Verification items for the finished model (mm, model axes). Face numbers are marked on the shaded views. Coordinates: 2 decimals unless noted, no trailing zeros. Loops run counter-clockwise (first coordinate to the right, second up) from the corner with the lowest first, then second, coordinate; pieces in that order, holes last. Notation, with made-up numbers: (32.25, 19.25) -> (52.25, 19.25) arc R26 ccw to (52.25, 55.25) -> close; hole circle Ø6 at (26.5, 27.25). An arc over 180 degrees is marked (long way). Write item = value, one per line.
```python
from build123d import *

# Parameters (mm, degrees)
F0_W     = 50
F0_H     = 48
F1_DEPTH = 20
F2_R     = 24.99999
F3_R     = 12.5
F4_DEPTH = 25


# Not quite as in the source:
# - a fillet or chamfer is up to 0.001 mm smaller than in the source, because OpenCascade refuses the exact size


with BuildPart() as f1:
    # F0 (on Front) → F1 (new body)
    with BuildSketch(Plane.XZ):
        with Locations((-20.5971896648, 6.0340394775)):
            Rectangle(F0_W, F0_H)
    extrude(amount=F1_DEPTH)

    # F2 (radius 25 in the source; OpenCascade refuses exactly that, so slightly less here)
    f2_edges = [f1.edges().sort_by_distance(p)[0] for p in [
        (4.40281, -10, 30.034039),
        (-45.59719, -10, 30.034039),
    ]]
    fillet(f2_edges, radius=F2_R)

    # F3 (on face) → F4 (cut)
    with BuildSketch(Plane(origin=(0, 0, 0), x_dir=(-1, 0, 0), z_dir=(0, 1, 0))):
        with Locations((20.5971896648, 5.0340394775)):
            Circle(F3_R)
    extrude(amount=-F4_DEPTH, mode=Mode.SUBTRACT)


solid = f1.part
```
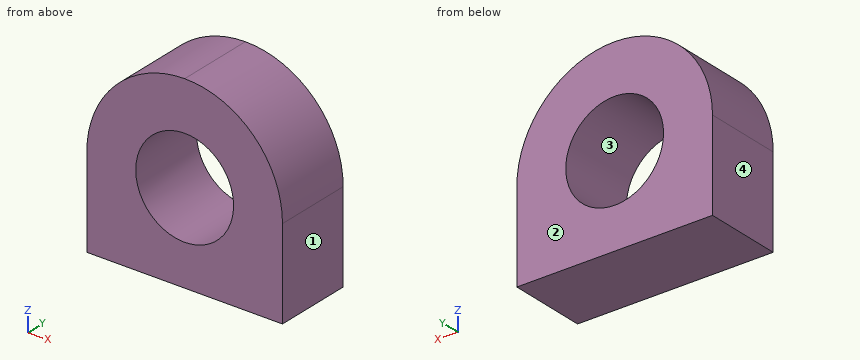
1) Release check for a two-part mould opening along X. For the marked faces 1, 2, 3 and 4 record: pulls with the +X half, pulls with the -X half, needs draft (parallel to the pull), parting line crosses it, or undercut.
Ans:
face_1 = pulls with the +X half
face_2 = needs draft
face_3 = undercut
face_4 = pulls with the -X half
2) Sectioned sample at A-A, the plane x = -15.5. Record the cut outline in (y, z).
Ans:
outline = (-20, -17.97) -> (0, -17.97) -> (0, -6.38) -> (-20, -6.38) -> close; (-20, 16.45) -> (0, 16.45) -> (0, 29.51) -> (-20, 29.51) -> close
3) Sectioned sample at D-D, the plane x = -34.5. Record the cut outline in (y, z), plus the area to 3 significant figures.
Ans:
outline = (-20, -17.97) -> (0, -17.97) -> (0, 25.81) -> (-20, 25.81) -> close
area = 876 mm2
4) Sectioned sample at B-B, the plane z = 9.5. Record the cut outline in (x, y), plus the area to 3 significant figures.
Ans:
outline = (-45.2, -20) -> (-32.27, -20) -> (-32.27, 0) -> (-45.2, 0) -> close; (-8.92, -20) -> (4, -20) -> (4, 0) -> (-8.92, 0) -> close
area = 517 mm2
5) Material ranges on line 1 (Z direction, x = -20, y = -6); line 2 (Z direction, x = -25.5, y = -3.25); line 3 (X direction, y = -2.25, z = 6.5), recorded low to high.
Ans:
line_1 = -17.97 to -7.45, 17.52 to 30.03
line_2 = -17.97 to -6.46, 16.53 to 29.55
line_3 = -45.55 to -33.01, -8.18 to 4.36
6) Depth check by flat-ended pin: pin 1 Ø6 at (x, y) = (-17.5, -8) entering from +Z; pin 2 Ø4 at (y, z) = (-17.5, 21.5) entering from +X. Enter the tip coordinate at first touch or a pass-through.
Ans:
pin_1 = 30.03
pin_2 = -0.21
